Autodesk Inventor part; units mm, degrees
ref_plane "YZ Plane" through (0, 0, 0) normal (1, 0, 0) x (0, 1, 0)
ref_plane "XZ Plane" through (0, 0, 0) normal (0, 1, 0) x (-1, 0, 0)
ref_plane "XY Plane" through (0, 0, 0) normal (0, 0, 1) x (1, 0, 0)
sketch "Boceto1" plane through (0, 0, 0) normal (0, 0, 1) x (1, 0, 0)
  line L0 (-400, 800) -> (400, 800)
  line L1 (400, 800) -> (400, 0)
  line L2 (400, 0) -> (-400, 0)
  line L3 (-400, 0) -> (-400, 800)
  circle A0 centre (0, 400) radius 283.4638
  line L4 (-400, 400) -> (400, 400)
  point P0 (0, 0)
  point P1 (0, 0)
  dimension "d0" = 800
extrude "Extrusión1" add sketch "Boceto1" along normal blind 150 contours L0 L1 L4 A0 L3 | L4 A0 L1 L2 L3
properties part number "Bobina"
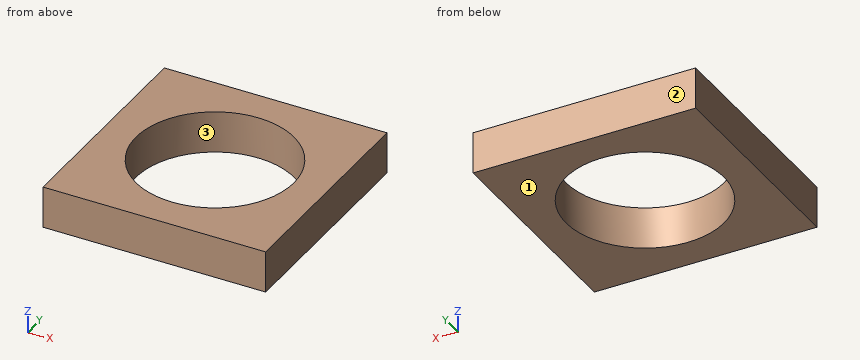
Model file for the job. Use its own axes, mm. Face numbers are marked on the shaded views. Give positions to 0.01 mm unless a question says otherwise; leave off trailing zeros. Write each loop counter-clockwise with the first axis right and the second up, starting at its lowest first coordinate (ties: lowest second). Pieces come first, ordered by that corner, then holes. Notation, with made-up numbers: (-9.5, 14.5) - (48.5, 14.5) arc R22 cw to (48.5, 39.5) - close; hole circle Ø2 at (2.5, 30.5). An arc over 180 degrees is marked (long way). One line per question, with ' | ' between items. Start each with the question number.
(1) Wall check: line 1 along X through (y, z) = (400, 72); line 2 along Y through (x, z) = (0, 41); line 3 along Y through (x, z) = (-72, 76). Give the ranges that are in metal, low to high. Write a range as from..to.
(2) Two-plate mould, pull along Y, no slides. Class the marked faces 1, 2 and 3: +Y half, -Y half, draft (parallel to the pull), parting line (faces both ways), or undercut.
(3) Slice it at B-B on z = 138. Write the cut outline in (x, y).
(4) Slice it at A-A on x = 0. Write the cut outline in (y, z), plus the area to 3 significant figures.
(5) Slice it at C-C on y = 400. Write the cut outline in (x, z), plus the area to 3 significant figures.
Results below:
1) line 1: -400..-283.46, 283.46..400 | line 2: 0..116.54, 683.46..800 | line 3: 0..125.83, 674.17..800
2) face 1: draft | face 2: +Y half | face 3: undercut
3) outline: (-400, 0) - (400, 0) - (400, 800) - (-400, 800) - close; hole circle Ø566.93 at (0, 400)
4) outline: (0, 0) - (116.54, 0) - (116.54, 150) - (0, 150) - close; (683.46, 0) - (800, 0) - (800, 150) - (683.46, 150) - close | area: 35,000 mm^2
5) outline: (-400, 0) - (-283.46, 0) - (-283.46, 150) - (-400, 150) - close; (283.46, 0) - (400, 0) - (400, 150) - (283.46, 150) - close | area: 35,000 mm^2
